```python
from build123d import *

# Parameters (mm, degrees)
F0_R     = 1.2331232955
F0_R_2   = 1.2314274958
F1_DEPTH = 2.9718


# Not quite as in the source:
# - a feature names something its author has since deleted; it is built from what else it names


with BuildPart() as f1:
    # F0 (on Right) → F1 (new body)
    with BuildSketch(Plane.YZ):
        with BuildLine():
            Line((-31.8963663923, 52.0706325769), (-31.8963663923, 69.3939922799))
            Line((-31.8963663923, 69.3939922799), (-36.9763663923, 69.3939922799))
            Line((-36.9763663923, 69.3939922799), (-38.147252053, 69.3939922799))
            Line((-38.147252053, 69.3939922799), (-38.147252053, 72.360080524))
            Line((-38.147252053, 72.360080524), (-57.2884293294, 72.360080524))
            Line((-57.2884293294, 72.360080524), (-57.2884293294, 69.3939922799))
            Line((-57.2884293294, 69.3939922799), (-72.6028546119, 69.3939922799))
            Line((-72.6028546119, 69.3939922799), (-72.6028546119, 72.360080524))
            Line((-72.6028546119, 72.360080524), (-92.9228546119, 72.360080524))
            Line((-92.9228546119, 72.360080524), (-92.9228546119, 69.3939922799))
            Line((-92.9228546119, 69.3939922799), (-108.1628546119, 69.3939922799))
            Line((-108.1628546119, 69.3939922799), (-108.1628546119, 18.7421012782))
            ThreePointArc((-108.1628546119, 18.7421012782), (-107.6580863604, 16.2610196982), (-106.2240307358, 14.1743857437))
            Line((-106.2240307358, 14.1743857437), (-31.8963663923, -57.6060077201))
            Line((-31.8963663923, -57.6060077201), (-31.8963663923, -16.9660077201))
            Line((-31.8963663923, -16.9660077201), (-31.8967170966, -14.0375348575))
            Line((-31.8967170966, -14.0375348575), (-28.9245663923, -14.0371789226))
            Line((-28.9245663923, -14.0371789226), (-28.9245663923, 3.3539922799))
            Line((-28.9245663923, 3.3539922799), (-28.9245663923, 6.2467521057))
            Line((-28.9245663923, 6.2467521057), (-31.8963663923, 6.2467521057))
            Line((-31.8963663923, 6.2467521057), (-31.988988285, 17.581195007))
            Line((-31.988988285, 17.581195007), (-37.0603909409, 17.581195007))
            Line((-37.0603909409, 17.581195007), (-37.0603909409, 15.8720928303))
            Line((-37.0603909409, 15.8720928303), (-39.6003909409, 15.8720928303))
            Line((-39.6003909409, 15.8720928303), (-39.6003909409, 17.581195007))
            Line((-39.6003909409, 17.581195007), (-44.6717935968, 17.581195007))
            Line((-44.6717935968, 17.581195007), (-44.6717935968, 20.5129906535))
            Line((-44.6717935968, 20.5129906535), (-39.6003909409, 20.5129906535))
            Line((-39.6003909409, 20.5129906535), (-39.6003909409, 22.2220928303))
            Line((-39.6003909409, 22.2220928303), (-37.0603909409, 22.2220928303))
            Line((-37.0603909409, 22.2220928303), (-37.0603909409, 20.5129906535))
            Line((-37.0603909409, 20.5129906535), (-31.988988285, 20.5129906535))
            Line((-31.988988285, 20.5129906535), (-32.0563334468, 28.7542376011))
            Line((-32.0563334468, 28.7542376011), (-32.0563334468, 31.9596784297))
            Line((-32.0563334468, 31.9596784297), (-29.0845334468, 31.9596784297))
            Line((-29.0845334468, 31.9596784297), (-29.0845334468, 49.0742376011))
            Line((-29.0845334468, 49.0742376011), (-29.0845334468, 52.0706325769))
            Line((-29.0845334468, 52.0706325769), (-31.8963663923, 52.0706325769))
        make_face()
        with Locations((-30.6644663923, -6.7510945896)):
            Circle(F0_R, mode=Mode.SUBTRACT)
        with Locations((-82.6862763941, 70.623036402)):
            Circle(F0_R_2, mode=Mode.SUBTRACT)
        with BuildLine():
            ThreePointArc((-29.4325663923, 42.0150328428), (-30.6644663923, 40.7831328428), (-31.8963663923, 42.0150328428))
            ThreePointArc((-31.8963663923, 42.0150328428), (-30.6644663923, 43.2469328428), (-29.4325663923, 42.0150328428))
        make_face(mode=Mode.SUBTRACT)
        with Locations((-47.2050075472, 70.623036402)):
            Circle(F0_R_2, mode=Mode.SUBTRACT)
    extrude(amount=F1_DEPTH)


solid = f1.part
```
Geometry check sheet. Reference: the model listing, model coordinates, mm. A direction names the side the tool comes from. Coordinates: 2 decimals unless noted, no trailing zeros. Loops run counter-clockwise (first coordinate to the right, second up) from the corner with the lowest first, then second, coordinate; pieces in that order, holes last.
Item 1: Sectioned sample at B-B, the plane z = 60.5. Record the boundary of the cut face in (x, y).
Item 2: Access from +Z, -Z, +X, -X, +Y, -Y to the whole of each face (thin tool, end or side, straight path). Record for faces 1 (the face through (1, -38.147, 71)), 2 (the face through (1, -108.163, 44)), 3 (the face through (1, -42, 20.513)), 4 (the face through (1, -65, 69.394)), 5 (the face through (1, -83, 72.36)).
Item 3: Sectioned sample at D-D, the plane x = 0.5. Count the separate pieces of the cut face and the enclosed holes in it, then the cut area to 3 significant figures.
Item 4: Thickness scan on line 1 (Y direction, x = 0.25, z = 21.5); line 2 (Z direction, x = 0.45, y = -98); line 3 (Y direction, x = 0.5, z = 33). Record the ranges inside material, lowest first.
Item 5: Sectioned sample at A-A, the plane y = -43. Record the boundary of the cut face in (x, z).
Item 6: Sectioned sample at C-C, the plane y = -34. Record the boundary of the cut face in (x, z).
Item 7: Go/stop test with flat-tipped pins: pin 1 Ø1.4 at (x, y) = (1.5, -30) entering from +Z; pin 2 Ø0.5 at (x, z) = (2, 17) entering from +Y; pin 3 Ø1.5 at (y, z) = (-30.66, 42.02) entering from +X; pin 4 Ø1.5 at (x, y) = (1, -43) entering from -Z. Record where each tip stops, or that it passes through.
Item 8: Release check for a two-part mould opening along Y. For faces 6 (the face through (0, -60, 23)), 7 (the face through (1.47, -29.49, -6.38)), 8 (the face through (1.47, -107.67, 16.29)) record: released by +Y, released by -Y, zero draft, split by the parting line, or undercut.
Check result:
1. outline: (0, -108.16) - (2.97, -108.16) - (2.97, -31.9) - (0, -31.9) - close
2. face 1: +Z, +X, -X, +Y
2. face 2: +Z, -Z, +X, -X, -Y
2. face 3: +X, -X, +Y
2. face 4: +Z, +X, -X
2. face 5: +Z, +X, -X, +Y, -Y
3. separate pieces: 1
3. enclosed holes: 4
3. area: 7,040 mm2
4. line 1: y = -108.16 to -39.6, -37.06 to -32
4. line 2: z = 6.23 to 69.39
4. line 3: y = -108.16 to -29.08
5. outline: (0, -46.88) - (2.97, -46.88) - (2.97, 17.58) - (0, 17.58) - close; (0, 20.51) - (2.97, 20.51) - (2.97, 72.36) - (0, 72.36) - close
6. outline: (0, -55.57) - (2.97, -55.57) - (2.97, 17.58) - (0, 17.58) - close; (0, 20.51) - (2.97, 20.51) - (2.97, 69.39) - (0, 69.39) - close
7. pin 1: stops at z = 52.07
7. pin 2: stops at y = -31.98
7. pin 3: passes through
7. pin 4: stops at z = -47.61
8. face 6: zero draft
8. face 7: undercut
8. face 8: released by -Y
